Autodesk Inventor part; units mm, degrees
ref_plane "Work Plane1" through (-4.5, 0, -1.5) normal (0, 1, 0) x (1, 0, 0)
ref_plane "YZ Plane" through (0, 0, 0) normal (1, 0, 0) x (0, 1, 0)
ref_plane "XZ Plane" through (0, 0, 0) normal (0, 1, 0) x (-1, 0, 0)
sketch "Sketch_1" plane through (0, 0, 0) normal (0, 0, 1) x (1, 0, 0)
  line L0 (-4.5, 4.5) -> (-4.5, -4.5)
  line L1 (-4.5, -4.5) -> (4.5, -4.5)
  line L2 (4.5, -4.5) -> (4.5, 4.5)
  line L3 (4.5, 4.5) -> (-4.5, 4.5)
extrude "Extrusion1" add sketch "Sketch_1" along normal mid plane 3
sketch "Sketch_2" plane through (0, 0, 0) normal (1, 0, 0) x (0, 1, 0)
  line L0 (0, -1.5) -> (0, 1.5)
  line L1 (0, 1.5) -> (2.5, 1.5)
  line L2 (2.5, 1.5) -> (2.067, 1.067)
  line L3 (2.067, 1.067) -> (2.067, -1.067)
  line L4 (2.067, -1.067) -> (2.5, -1.5)
  line L5 (2.5, -1.5) -> (0, -1.5)
  line L6 (0, -1.5) -> (0, 1.5)
revolve "Revolution1" cut sketch "Sketch_2" angle 360 about axis through (0, 0, -1.5) along (0, 0, -1)
thread "Thread1"
sketch "Sketch_3" plane through (0, 0, 0) normal (0, 1, 0) x (-1, 0, 0)
  line L0 (4.5, 0.5) -> (4.5, 2.5)
  line L1 (4.5, 2.5) -> (-4.5, 2.5)
  line L2 (-4.5, 2.5) -> (-4.5, 0.5)
  line L3 (-4.5, 0.5) -> (-3.5, 1.5)
  line L4 (-3.5, 1.5) -> (3.5, 1.5)
  line L5 (3.5, 1.5) -> (4.5, 0.5)
extrude "Extrusion2" cut sketch "Sketch_3" along normal mid plane 18
ref_plane "Work Plane1" through (-4.5, 0, -1.5) normal (0, 1, 0) x (1, 0, 0)
properties part number "T-Nut Block M5  Threads"
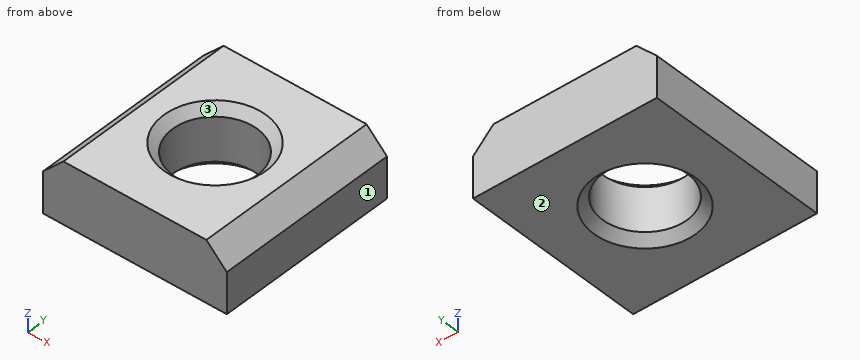
Can you work these out from the model? Positions are in its coordinate system, mm. Face numbers are marked on the shaded views. Coordinates: 2 decimals unless noted, no trailing zeros. Write each loop counter-clockwise with the first axis right and the second up, starting at its lowest first coordinate (ties: lowest second). Pieces come first, ordered by that corner, then holes. Notation, with made-up numbers: M 11.25,55 L 45.25,55 A6 ccw 45.25,63 Z; hole C 77.5,39 d2. An arc over 180 degrees is marked long. Answer as CSV lines item,"result".
Item 1: We'd pull the mould along X, two halves only. Please class the marked faces 1, 2 and 3: +X half, -X half, draft (parallel to the pull), parting line (faces both ways), or undercut.
Geometry results:
face 1,"+X half"
face 2,"draft"
face 3,"undercut"
Item 2: Imagine slicing it at B-B on y = 0. List the corners of the cut face in (x, z) for me.
Geometry results:
outline,"M -4.5,-1.5 L -2.5,-1.5 L -2.07,-1.07 L -2.07,1.07 L -2.5,1.5 L -3.5,1.5 L -4.5,0.5 Z; M 2.07,-1.07 L 2.5,-1.5 L 4.5,-1.5 L 4.5,0.5 L 3.5,1.5 L 2.5,1.5 L 2.07,1.07 Z"
Item 3: Imagine slicing it at A-A on x = 0. List the corners of the cut face in (y, z) for me, plus the area to 3 significant figures.
Geometry results:
outline,"M -4.5,-1.5 L -2.5,-1.5 L -2.07,-1.07 L -2.07,1.07 L -2.5,1.5 L -4.5,1.5 Z; M 2.07,-1.07 L 2.5,-1.5 L 4.5,-1.5 L 4.5,1.5 L 2.5,1.5 L 2.07,1.07 Z"
area,"14.2 mm2"
Item 4: Imagine slicing it at C-C on z = 1.3. List the corners of the cut face in (x, y) for me.
Geometry results:
outline,"M -3.7,-4.5 L 3.7,-4.5 L 3.7,4.5 L -3.7,4.5 Z; hole C 0,0 d4.6"
Item 5: I'm going to push a flat-ended pin straight in: P1, Ø1.5, axis at x = -1, y = 2, coming from the +Z side. Where does the tip first touch, or does it pass through?
Geometry results:
P1,"stops at z = 1.5"
Item 6: Please list where these lines run through material, in increasing order: line 1 along X through (y, z) = (0, -0.1); line 2 along X through (y, z) = (0, 0.65); line 3 along X through (y, z) = (-3.5, 1.2).
Geometry results:
line 1,"x = -4.5 to -2.07, 2.07 to 4.5"
line 2,"x = -4.35 to -2.07, 2.07 to 4.35"
line 3,"x = -3.8 to 3.8"
